Source: three-view drawing plus pictorial views. Frame: mm from the lowest corner of the part. A direction names the side the tool comes from. Round coordinates to 2 decimals unless told otherwise and drop trailing zeros. Loops run counter-clockwise (first coordinate to the right, second up) from the corner with the lowest first, then second, coordinate; pieces in that order, holes last. Notation, with made-up numbers: (3.5, 83) -> (15.5, 83) arc R7 ccw to (15.5, 92) -> close; hole circle Ø8 at (20, 50.25). An arc over 180 degrees is marked (long way). Put each result on its own line as item: value. Start each with the question number.
1. Set-up query: the marked faces 1, 2, 3 and 4. Return all of +Z, -Z, +X, -X, +Y, -Y with unobstructed straight access to the full face (end or side cutting, diameter ignored); none if empty.
2. Cut plane B-B (x = 10). Return the cut outline in (y, z).
3. Cut plane D-D (z = 12). Return the cut outline in (x, y).
4. Cut plane C-C (y = 37.5). Return the cut outline in (x, z), then the cut area to 3 significant figures.
5. Material intervals for L1, parallel to Y at x = 5, z = 15.4; L2, parallel to Y at x = 8.75, z = 25.5; L3, parallel to Z at x = 5.5, y = 18, sorted ascending.
6. Contact query for flat-ended pins moving along their axis: pin 1 (6 mm diameter, centred on x = 10, y = 50.5, fed in from -Z); pin 2 (2 mm diameter, centred on x = 12.5, y = 4.5, fed in from -Z); pin 3 (6 mm diameter, centred on x = 5, y = 3.4, fed in from +Z). Output: stop coordinate, or through.
7. Cut plane A-A (y = 3.4). Return the cut outline in (x, z), then the cut area to 3 significant figures.
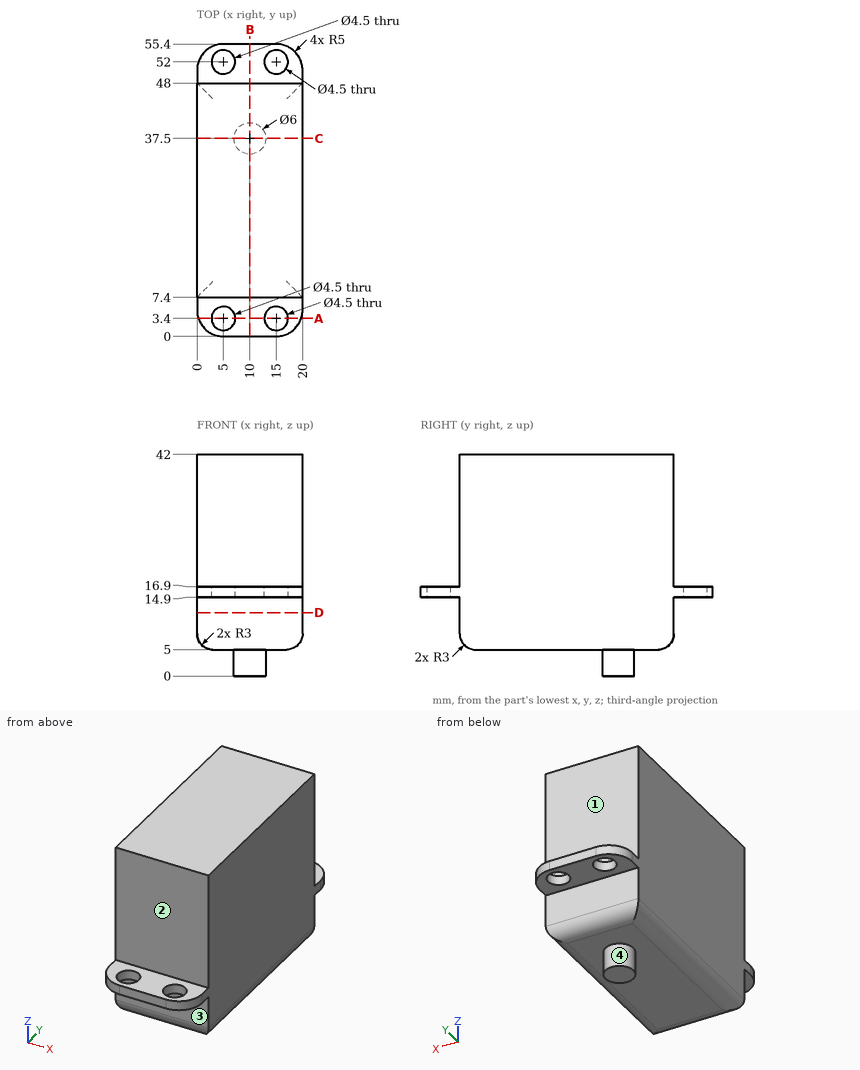
Solution:
1. face 1: +Z, +X, -X, +Y
1. face 2: +Z, +X, -X, -Y
1. face 3: -Z, +X, -X, -Y
1. face 4: -Z
2. outline: (0, 14.9) -> (7.4, 14.9) -> (7.4, 8) arc R3 ccw to (10.4, 5) -> (34.5, 5) -> (34.5, 0) -> (40.5, 0) -> (40.5, 5) -> (45, 5) arc R3 ccw to (48, 8) -> (48, 14.9) -> (55.4, 14.9) -> (55.4, 16.9) -> (48, 16.9) -> (48, 42) -> (7.4, 42) -> (7.4, 16.9) -> (0, 16.9) -> close
3. outline: (0, 7.4) -> (20, 7.4) -> (20, 48) -> (0, 48) -> close
4. outline: (0, 8) arc R3 ccw to (3, 5) -> (7, 5) -> (7, 0) -> (13, 0) -> (13, 5) -> (17, 5) arc R3 ccw to (20, 8) -> (20, 42) -> (0, 42) -> close
4. area: 766 mm^2
5. L1: y = 0 to 1.15, 5.65 to 49.75, 54.25 to 55.4
5. L2: y = 7.4 to 48
5. L3: z = 5 to 42
6. pin 1: stops at z = 6.34
6. pin 2: stops at z = 14.9
6. pin 3: stops at z = 16.9
7. outline: (0.26, 14.9) -> (2.75, 14.9) -> (2.75, 16.9) -> (0.26, 16.9) -> close; (7.25, 14.9) -> (12.75, 14.9) -> (12.75, 16.9) -> (7.25, 16.9) -> close; (17.25, 14.9) -> (19.74, 14.9) -> (19.74, 16.9) -> (17.25, 16.9) -> close
7. area: 20.9 mm^2
